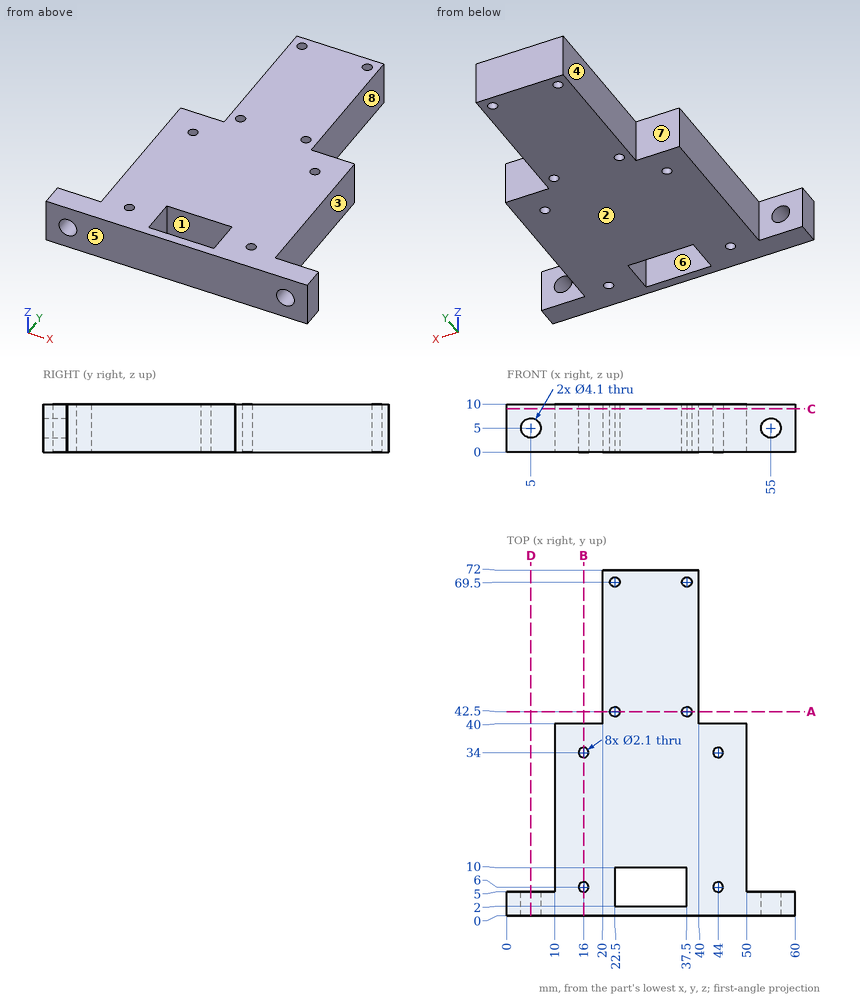
Here's the drawing with two shaded views (mm, measured from the low corner). I have some questions. A direction names the side the tool comes from. Coordinates: 2 decimals unless noted, no trailing zeros. Loops run counter-clockwise (first coordinate to the right, second up) from the corner with the lowest first, then second, coordinate; pieces in that order, holes last. Notation, with made-up numbers: (24, 5) - (73, 5) arc R20 cw to (73, 22) - close; hole circle Ø1 at (82.5, -12.5). An arc over 180 degrees is marked (long way). Answer as CSV lines item,"result". Start each with the question number.
1) Suppose I cut it at A-A (y = 42.5). Please give me the cut outline in (x, z), plus the area to 3 significant figures.
2) Suppose I cut it at D-D (x = 5). Please give me the cut outline in (y, z), plus the area to 3 significant figures.
3) Thinking about a two-plate mould opening in X: for the marked faces 6, 7 and 8, which applies, pulls with the +X half, pulls with the -X half, needs draft (parallel to the pull), parting line crosses it, or undercut?
4) For pin 1 (2 mm diameter, centred on y = 17, z = 9, fed in from -X); pin 2 (6 mm diameter, centred on y = 61, z = 4.5, fed in from -X); pin 3 (1.3 mm diameter, centred on x = 16, y = 34, fed in from -Z); pin 4 (5 mm diameter, centred on y = 59, z = 6, fed in from +X), each with a flat end and sliding along its axis, tell me the tip position at first contact or that it passes through.
5) Suppose I cut it at C-C (z = 9). Count the separate pieces of the cut face and the enclosed holes in it, plus the area to 3 significant figures.
6) Which directions (+Z, -Z, +X, -X, +Y, -Y) give clear straight access to the entire face, cutting with the end or side of a thin tool? Please do the marked faces 1, 2, 3, 4 and 5.
7) I need wall thicknesses on line 1 (Y direction, x = 44, z = 3.5); line 2 (X direction, y = 69.5, z = 7.75); line 3 (X direction, y = 69, z = 7.5). Which ranges of each line are inside material? Lowest first, please. Write a range as from..to.
8) Suppose I cut it at B-B (x = 16). Please give me the cut outline in (y, z).
Check result:
1,outline,"(20, 0) - (21.45, 0) - (21.45, 10) - (20, 10) - close; (23.55, 0) - (36.45, 0) - (36.45, 10) - (23.55, 10) - close; (38.55, 0) - (40, 0) - (40, 10) - (38.55, 10) - close"
1,area,"158 mm²"
2,outline,"(0, 0) - (5, 0) - (5, 2.95) - (0, 2.95) - close; (0, 7.05) - (5, 7.05) - (5, 10) - (0, 10) - close"
2,area,"29.5 mm²"
3,face 6,"undercut"
3,face 7,"needs draft"
3,face 8,"pulls with the +X half"
4,pin 1,"stops at x = 10"
4,pin 2,"stops at x = 20"
4,pin 3,"passes through"
4,pin 4,"stops at x = 40"
5,separate pieces,"1"
5,enclosed holes,"9"
5,area,"2,190 mm²"
6,face 1,"+Z, -Z"
6,face 2,"-Z, +X, -X, +Y, -Y"
6,face 3,"+Z, -Z, +X, +Y"
6,face 4,"+Z, -Z, -X, +Y"
6,face 5,"+Z, -Z, +X, -X, -Y"
7,line 1,"y = 0..4.95, 7.05..32.95, 35.05..40"
7,line 2,"x = 20..21.45, 23.55..36.45, 38.55..40"
7,line 3,"x = 20..21.58, 23.42..36.58, 38.42..40"
8,outline,"(0, 0) - (4.95, 0) - (4.95, 10) - (0, 10) - close; (7.05, 0) - (32.95, 0) - (32.95, 10) - (7.05, 10) - close; (35.05, 0) - (40, 0) - (40, 10) - (35.05, 10) - close"
